```python
from build123d import *

# Parameters (mm, degrees)
CROQUIS1_R                   = 1
SALIENTE_EXTRUIR1_DEPTH      = 20
SALIENTE_EXTRUIR1_DEPTH_BACK = 20
CROQUIS3_R                   = 1.5
CORTAR_EXTRUIR1_DEPTH        = 20
CROQUIS4_R                   = 2
CORTAR_EXTRUIR2_DEPTH        = 1.5


with BuildPart() as part:
    # Croquis1 → Saliente-Extruir1 (new body, two sides)
    with BuildSketch(Plane(origin=(0, 0, 0), x_dir=(0, 0, -1), z_dir=(1, 0, 0))) as saliente_extruir1_sk:
        with BuildLine():
            Line((-0.75, -12.7), (0.75, -12.7))
            Line((0.75, -12.7), (0.75, 12.7))
            Line((0.75, 12.7), (0.75, 14.2))
            ThreePointArc((0.75, 14.2), (-1.810660172, 15.260660172), (-0.75, 12.7))
            Line((-0.75, 12.7), (-0.75, -12.7))
        make_face()
        with Locations((-0.75, 14.2)):
            Circle(CROQUIS1_R, mode=Mode.SUBTRACT)
    extrude(amount=SALIENTE_EXTRUIR1_DEPTH)
    extrude(saliente_extruir1_sk.sketch, amount=-SALIENTE_EXTRUIR1_DEPTH_BACK)

    # Croquis3 → Cortar-Extruir1 (cut)
    with BuildSketch(Plane(origin=(20, 0, 0), x_dir=(0, 0, -1), z_dir=(1, 0, 0))):
        with Locations((-0.75, 14.2)):
            Circle(CROQUIS3_R)
    extrude(amount=-CORTAR_EXTRUIR1_DEPTH, mode=Mode.SUBTRACT)

    # Croquis4 → Cortar-Extruir2 (cut)
    with BuildSketch(Plane.XY.offset(0.75)):
        with Locations((-11.5, 0)):
            Circle(CROQUIS4_R)
        with Locations((11.5, 0)):
            Circle(CROQUIS4_R)
    extrude(amount=-CORTAR_EXTRUIR2_DEPTH, mode=Mode.SUBTRACT)


solid = part.part
```
Read the model definition and answer for the solid it produces. Units are mm, in the model's axes. A direction names the side the tool comes from. Coordinates: 2 decimals unless noted, no trailing zeros. Loops run counter-clockwise (first coordinate to the right, second up) from the corner with the lowest first, then second, coordinate; pieces in that order, holes last.
(1) A tool of negligible diameter and unlimited length cuts with its end or side. For faces 5 (the face through (0, -12.7, 0)), 6 (the face through (0, 0, 0.75)), from which of +Z, -Z, +X, -X, +Y, -Y can it reach the whole face along a straight path? Write none if from no direction.
Solution:
face 5: +Z, -Z, +X, -X, -Y
face 6: +Z, +X, -X, -Y
(2) The part is cut by section C-C (z = 1.35). Determine the outline of the cut face in (x, y), and give its area (3 significant figures).
Solution:
outline: (-20, 12.83) - (0, 12.83) - (0, 13.4) - (-20, 13.4) - close; (-20, 15) - (0, 15) - (0, 15.57) - (-20, 15.57) - close
area: 23.0 mm2
(3) The part is cut by section A-A (x = -11.5). Determine the outline of the cut face in (y, z), and give its area (3 significant figures).
Solution:
outline: (-12.7, -0.75) - (-2, -0.75) - (-2, 0.75) - (-12.7, 0.75) - close; (2, -0.75) - (14.2, -0.75) arc R1.5 ccw (long way) to (12.7, 0.75) - (2, 0.75) - close; hole circle Ø2 at (14.2, 0.75)
area: 36.5 mm2
(4) Flat-ended cylindrical pins translate along their axes: pin 1 Ø5 at (x, y) = (10, 9.5) entering from +Z; pin 2 Ø3 at (x, y) = (-11.5, 0) entering from +Z; pin 3 Ø12.5 at (x, y) = (1, 3) entering from +Z; pin 4 Ø0.9 at (y, z) = (14.5, 1.5) entering from +X. Find the tip coordinate at first contact, or state that the pin passes through.
Solution:
pin 1: stops at z = 0.75
pin 2: passes through
pin 3: stops at z = 0.75
pin 4: stops at x = 0
(5) The part is cut by section B-B (y = 0). Determine the outline of the cut face in (x, z), and give its area (3 significant figures).
Solution:
outline: (-20, -0.75) - (-13.5, -0.75) - (-13.5, 0.75) - (-20, 0.75) - close; (-9.5, -0.75) - (9.5, -0.75) - (9.5, 0.75) - (-9.5, 0.75) - close; (13.5, -0.75) - (20, -0.75) - (20, 0.75) - (13.5, 0.75) - close
area: 48.0 mm2
(6) The mould has two halves that part along X. Classify faces 1 (the face through (-13.1, -1.2, 0)), 2 (the face through (0, 13, 1)), 3 (the face through (9.502, 0.088, 0.01)), 4 (the face through (10.14, 13.13, -0.3)): released by +X, released by -X, zero draft, split by the parting line, or undercut.
Solution:
face 1: undercut
face 2: released by +X
face 3: undercut
face 4: zero draft
(7) Consider line 1 along Z through (x, y) = (8, 8.5); line 2 along Z through (x, y) = (-11, 13.75). Determine where each line is inside the solid, lowest interval first.
Solution:
line 1: z = -0.75 to 0.75
line 2: z = -0.75 to -0.14, 1.64 to 2.18
(8) The part is cut by section D-D (x = 11.5). Determine the outline of the cut face in (y, z).
Solution:
outline: (-12.7, -0.75) - (-2, -0.75) - (-2, 0.75) - (-12.7, 0.75) - close; (2, -0.75) - (14.2, -0.75) arc R1.5 cw to (12.7, 0.75) - (2, 0.75) - close
